Design review of the part shown in the three views and the two pictorial views. Dimensions are in mm from the part's minimum x, y and z. A direction names the side the tool comes from. Give positions to 0.01 mm unless a question says otherwise; leave off trailing zeros. Loops run counter-clockwise (first coordinate to the right, second up) from the corner with the lowest first, then second, coordinate; pieces in that order, holes last.
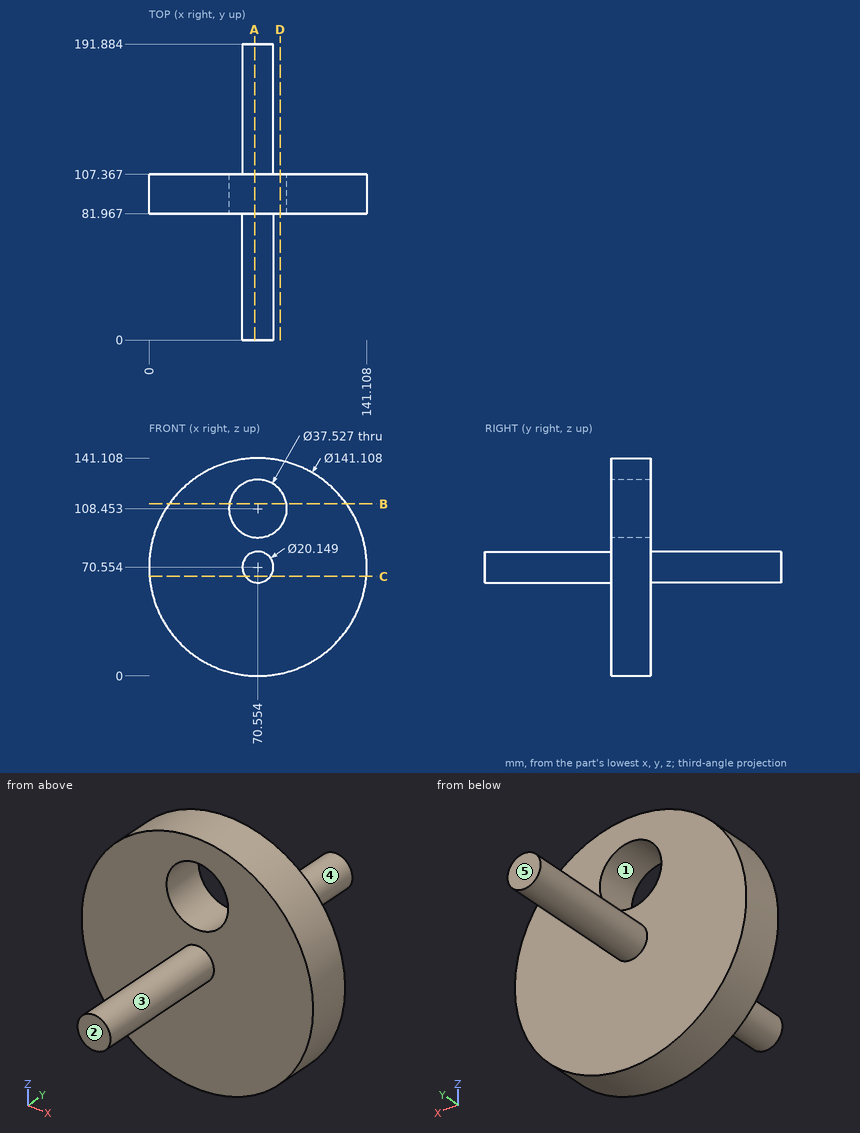
Q1. Take a section at D-D (x = 85). Give the boundary of the cut face in (y, z) (1 decimal), plus the area to 3 significant figures.
Results:
outline: (82, 1.5) - (107.4, 1.5) - (107.4, 96.5) - (82, 96.5) - close; (82, 120.4) - (107.4, 120.4) - (107.4, 139.6) - (82, 139.6) - close
area: 2,900 mm2
Q2. Insertion check: pin 1 (5 mm diameter, centred on y = 80.5, z = 81.5, fed in from +X); pin 2 (12 mm diameter, centred on x = 70.5, y = 65, fed in from +Z); pin 3 (8 mm diameter, centred on x = 109, z = 40.5, fed in from +Y). Each pin has a flat end and moves straight along its axis. Give the tip position at first contact, or say it passes through.
Results:
pin 1: stops at x = 140.54
pin 2: stops at z = 80.63
pin 3: stops at y = 107.37
Q3. Wall thickness on line 1 (Y direction, x = 26, z = 22.5); line 2 (Z direction, x = 97.5, y = 102.5); line 3 (X direction, y = 134, z = 73.5): over which ranges is each line inside the solid? List them lowest first.
Results:
line 1: y = 81.97 to 107.37
line 2: z = 5.35 to 135.76
line 3: x = 60.92 to 80.19
Q4. Draft analysis for pull direction X (two halves, no side actions). For the marked faces 1, 2 and 3, state which applies: pulls with the +X half, pulls with the -X half, needs draft (parallel to the pull), parting line crosses it, or undercut.
Results:
face 1: undercut
face 2: needs draft
face 3: parting line crosses it
Q5. Take a section at C-C (z = 64.5). Give the boundary of the cut face in (x, y).
Results:
outline: (0.26, 81.97) - (62.5, 81.97) - (62.5, 0) - (78.61, 0) - (78.61, 81.97) - (140.85, 81.97) - (140.85, 107.37) - (78.61, 107.37) - (78.61, 191.88) - (62.5, 191.88) - (62.5, 107.37) - (0.26, 107.37) - close
Q6. Take a section at B-B (z = 111.5). Give the boundary of the cut face in (x, y).
Results:
outline: (13.1, 81.97) - (52.04, 81.97) - (52.04, 107.37) - (13.1, 107.37) - close; (89.07, 81.97) - (128.01, 81.97) - (128.01, 107.37) - (89.07, 107.37) - close
Q7. Take a section at A-A (x = 68.5). Give the boundary of the cut face in (y, z).
Results:
outline: (0, 60.69) - (81.97, 60.69) - (81.97, 0.03) - (107.37, 0.03) - (107.37, 60.69) - (191.88, 60.69) - (191.88, 80.42) - (107.37, 80.42) - (107.37, 89.8) - (81.97, 89.8) - (81.97, 80.42) - (0, 80.42) - close; (81.97, 127.1) - (107.37, 127.1) - (107.37, 141.08) - (81.97, 141.08) - close
Q8. Tool access review of the marked faces 4 and 5: name each direction out of +Z, -Z, +X, -X, +Y, -Y from which nothing blocks a thin tool from reaching the whole face with its end or side.
Results:
face 4: +Y
face 5: +Z, -Z, +X, -X, +Y
